Model file for the job. Use its own axes, mm. Face numbers are marked on the shaded views. A direction names the side the tool comes from. Coordinates: 2 decimals unless noted, no trailing zeros. Order: outer loops, then holes, each group sorted by start corner. A loop starts at its lowest first (then second) coordinate and runs counter-clockwise, first axis right, second up. Notation, with made-up numbers: (54, 62) -> (68, 62) arc R21 ccw to (68, 78) -> close; hole circle Ø8 at (42.5, -1.5). An arc over 180 degrees is marked (long way). Use CSV: the item, a comma, the result in double quotes. Start each with the question number.
(1) Cut at C-C on y = -13.5. Write the cut outline in (x, z) (3 decimals).
(2) Cut at B-B on x = 27.5. Write the cut outline in (y, z), plus the area to 3 significant figures.
(3) Pin check, flat tips, straight feed: pin 1 Ø1.5 at (x, y) = (16, -82) entering from +Z; pin 2 Ø0.7 at (x, y) = (14, -82) entering from -Z; pin 3 Ø9.5 at (x, y) = (21.5, -32) entering from -Z. Stop position of each tip, or through.
(4) Probe L1, parallel to Y at x = 30, z = 11; L2, parallel to Y at x = 16, z = 21.5 (3 decimals); L3, parallel to X at y = 15.5, z = 12. List the from-to ranges inside material, lowest first.
(5) Tool access for the marked faces 1, 2 and 3: list every direction of +Z, -Z, +X, -X, +Y, -Y with a clear straight run to the whole face (end or side of a thin tool).
(6) Pull direction X, two halves, no side cores. Call the marked faces 4, 5 and 6: pulls with the +X half, pulls with the -X half, needs draft (parallel to the pull), parting line crosses it, or undercut.
(7) Cut at A-A on z = 14. Write the cut outline in (x, y) (3 decimals), plus the area to 3 significant figures.
(8) Cut at D-D on z = 2.5. Write the cut outline in (x, y).
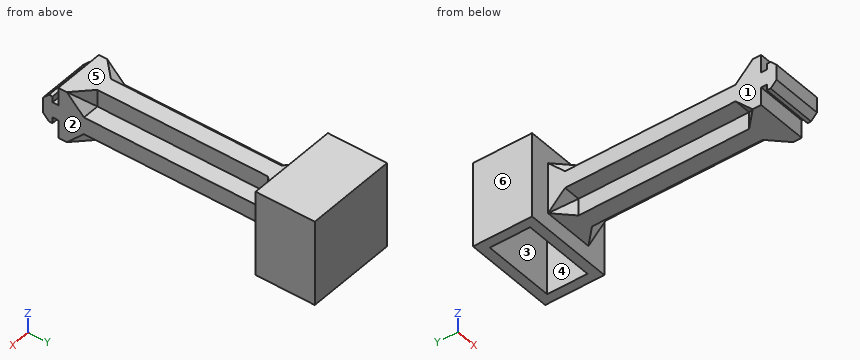
```python
from build123d import *

# Parameters (mm, degrees)
SKETCH1_W           = 34
SKETCH1_H           = 22
BOSS_EXTRUDE1_DEPTH = 31.75
SHELL1_T            = -3.5
BOSS_EXTRUDE2_DEPTH = 76.2
BOSS_EXTRUDE3_START = 26.525
BOSS_EXTRUDE3_DEPTH = 19.05
CHAMFER1_SIZE       = 6.35


with BuildPart() as part:
    # Sketch1 → Boss-Extrude1 (new body)
    with BuildSketch(Plane.XY):
        with Locations((17, 11)):
            Rectangle(SKETCH1_W, SKETCH1_H)
    extrude(amount=BOSS_EXTRUDE1_DEPTH)

    # Shell1
    shell1_openings = [part.faces().sort_by_distance(p)[0] for p in [
        (17, 11, 0),
    ]]
    offset(amount=SHELL1_T, openings=shell1_openings, kind=Kind.INTERSECTION)

    # Sketch2 → Boss-Extrude2 (add)
    with BuildSketch(Plane.XZ):
        Polygon((13.825, 25.189889706), (13.825, 18.839889706), (7.475, 18.839889706), (7.475, 12.489889706), (13.825, 12.489889706), (13.825, 6.139889706), (20.175, 6.139889706), (20.175, 12.489889706), (26.525, 12.489889706), (26.525, 18.839889706), (20.175, 18.839889706), (20.175, 25.189889706), align=None)
    extrude(amount=BOSS_EXTRUDE2_DEPTH)

    # Sketch3 → Boss-Extrude3 (add)
    with BuildSketch(Plane(origin=(0, 0, 0), x_dir=(0, 0, -1), z_dir=(1, 0, 0)).offset(BOSS_EXTRUDE3_START)):
        Polygon((-10.584889706, -81.534), (-10.584889706, -82.8675), (-12.807389706, -85.09), (-18.522389706, -85.09), (-20.744889706, -82.8675), (-20.744889706, -81.534), (-18.522389706, -81.534), (-18.522389706, -79.375), (-25.189889706, -79.375), (-25.189889706, -76.2), (-6.139889706, -76.2), (-6.139889706, -79.375), (-12.807389706, -79.375), (-12.807389706, -81.534), align=None)
    extrude(amount=-BOSS_EXTRUDE3_DEPTH)

    # Chamfer1
    # the kernel refuses this chamfer: 6.35 mm, written as the material it adds along each edge
    with BuildSketch(Plane(origin=(30.155186974, -76.2, 18.839889706), x_dir=(0, -0.027495876610585664, 0.9996219169112966), z_dir=(-1, 0, 0))) as chamfer1_piece_1_section:
        Polygon((CHAMFER1_SIZE * 0.999621916911, CHAMFER1_SIZE * 0.0274958766106), (-CHAMFER1_SIZE * 0.0274958766106, CHAMFER1_SIZE * 0.999621916911), (0, 0), align=None)
    chamfer1_piece_1 = extrude(amount=22.680186974, mode=Mode.PRIVATE)
    chamfer1_piece_1 = split(chamfer1_piece_1, bisect_by=Plane(origin=(26.525, -74.083333333, 20.956556373), z_dir=(-1, 0, 0)), keep=Keep.TOP, mode=Mode.PRIVATE)
    add(chamfer1_piece_1)
    with BuildSketch(Plane(origin=(13.825, -76.2, 25.189889706), x_dir=(-0.9996219169112966, -0.027495876610585654, 0), z_dir=(0, 0, -1))) as chamfer1_piece_2_section:
        Polygon((CHAMFER1_SIZE * 0.999621916911, CHAMFER1_SIZE * 0.0274958766106), (-CHAMFER1_SIZE * 0.0274958766106, CHAMFER1_SIZE * 0.999621916911), (0, 0), align=None)
    chamfer1_piece_2 = extrude(amount=22.680186974, mode=Mode.PRIVATE)
    chamfer1_piece_2 = split(chamfer1_piece_2, bisect_by=Plane(origin=(11.708333333, -74.083333333, 6.139889706), z_dir=(0, 0, 1)), keep=Keep.TOP, mode=Mode.PRIVATE)
    add(chamfer1_piece_2)
    with BuildSketch(Plane(origin=(26.525, -76.2, 18.839889706), x_dir=(0, -0.027495876610585654, 0.9996219169112968), z_dir=(-1, 0, 0))) as chamfer1_piece_3_section:
        Polygon((CHAMFER1_SIZE * 0.999621916911, CHAMFER1_SIZE * 0.0274958766106), (-CHAMFER1_SIZE * 0.0274958766106, CHAMFER1_SIZE * 0.999621916911), (0, 0), align=None)
    chamfer1_piece_3 = extrude(amount=22.680186974, mode=Mode.PRIVATE)
    chamfer1_piece_3 = split(chamfer1_piece_3, bisect_by=Plane(origin=(7.475, -74.083333333, 20.956556373), z_dir=(1, 0, 0)), keep=Keep.TOP, mode=Mode.PRIVATE)
    add(chamfer1_piece_3)
    with BuildSketch(Plane(origin=(20.175, -76.2, 2.509702732), x_dir=(0.9996219169112966, -0.02749587661058565, 0), z_dir=(0, 0, 1))) as chamfer1_piece_4_section:
        Polygon((CHAMFER1_SIZE * 0.999621916911, CHAMFER1_SIZE * 0.0274958766106), (-CHAMFER1_SIZE * 0.0274958766106, CHAMFER1_SIZE * 0.999621916911), (0, 0), align=None)
    chamfer1_piece_4 = extrude(amount=22.680186974, mode=Mode.PRIVATE)
    chamfer1_piece_4 = split(chamfer1_piece_4, bisect_by=Plane(origin=(22.291666667, -74.083333333, 6.139889706), z_dir=(0, 0, 1)), keep=Keep.TOP, mode=Mode.PRIVATE)
    add(chamfer1_piece_4)
    with BuildSketch(Plane(origin=(3.844813026, -76.2, 12.489889706), x_dir=(0, -0.027495876610585654, -0.9996219169112966), z_dir=(1, 0, 0))) as chamfer1_piece_5_section:
        Polygon((CHAMFER1_SIZE * 0.999621916911, CHAMFER1_SIZE * 0.0274958766106), (-CHAMFER1_SIZE * 0.0274958766106, CHAMFER1_SIZE * 0.999621916911), (0, 0), align=None)
    chamfer1_piece_5 = extrude(amount=22.680186974, mode=Mode.PRIVATE)
    chamfer1_piece_5 = split(chamfer1_piece_5, bisect_by=Plane(origin=(7.475, -74.083333333, 10.373223039), z_dir=(1, 0, 0)), keep=Keep.TOP, mode=Mode.PRIVATE)
    add(chamfer1_piece_5)
    with BuildSketch(Plane(origin=(20.175, -76.2, 6.139889706), x_dir=(0.9996219169112966, -0.02749587661058565, 0), z_dir=(0, 0, 1))) as chamfer1_piece_6_section:
        Polygon((CHAMFER1_SIZE * 0.999621916911, CHAMFER1_SIZE * 0.0274958766106), (-CHAMFER1_SIZE * 0.0274958766106, CHAMFER1_SIZE * 0.999621916911), (0, 0), align=None)
    chamfer1_piece_6 = extrude(amount=22.680186974, mode=Mode.PRIVATE)
    chamfer1_piece_6 = split(chamfer1_piece_6, bisect_by=Plane(origin=(22.291666667, -74.083333333, 25.189889706), z_dir=(0, 0, -1)), keep=Keep.TOP, mode=Mode.PRIVATE)
    add(chamfer1_piece_6)
    with BuildSketch(Plane(origin=(7.475, -76.2, 12.489889706), x_dir=(0, -0.027495876610585654, -0.9996219169112966), z_dir=(1, 0, 0))) as chamfer1_piece_7_section:
        Polygon((CHAMFER1_SIZE * 0.999621916911, CHAMFER1_SIZE * 0.0274958766106), (-CHAMFER1_SIZE * 0.0274958766106, CHAMFER1_SIZE * 0.999621916911), (0, 0), align=None)
    chamfer1_piece_7 = extrude(amount=22.680186974, mode=Mode.PRIVATE)
    chamfer1_piece_7 = split(chamfer1_piece_7, bisect_by=Plane(origin=(26.525, -74.083333333, 10.373223039), z_dir=(-1, 0, 0)), keep=Keep.TOP, mode=Mode.PRIVATE)
    add(chamfer1_piece_7)
    with BuildSketch(Plane(origin=(13.825, -76.2, 28.820076679), x_dir=(-0.9996219169112966, -0.02749587661058566, 0), z_dir=(0, 0, -1))) as chamfer1_piece_8_section:
        Polygon((CHAMFER1_SIZE * 0.999621916911, CHAMFER1_SIZE * 0.0274958766106), (-CHAMFER1_SIZE * 0.0274958766106, CHAMFER1_SIZE * 0.999621916911), (0, 0), align=None)
    chamfer1_piece_8 = extrude(amount=22.680186974, mode=Mode.PRIVATE)
    chamfer1_piece_8 = split(chamfer1_piece_8, bisect_by=Plane(origin=(11.708333333, -74.083333333, 25.189889706), z_dir=(0, 0, -1)), keep=Keep.TOP, mode=Mode.PRIVATE)
    add(chamfer1_piece_8)
    with BuildSketch(Plane(origin=(13.825, 0, 25.189889706), x_dir=(-0.9996219169112966, 0.02749587661058637, 0), z_dir=(0, 0, -1))) as chamfer1_piece_9_section:
        Polygon((CHAMFER1_SIZE * 0.999621916911, -CHAMFER1_SIZE * 0.0274958766106), (-CHAMFER1_SIZE * 0.0274958766106, -CHAMFER1_SIZE * 0.999621916911), (0, 0), align=None)
    chamfer1_piece_9 = extrude(amount=22.680186974, mode=Mode.PRIVATE)
    chamfer1_piece_9 = split(chamfer1_piece_9, bisect_by=Plane(origin=(11.708333333, -2.116666667, 6.139889706), z_dir=(0, 0, 1)), keep=Keep.TOP, mode=Mode.PRIVATE)
    add(chamfer1_piece_9)
    with BuildSketch(Plane(origin=(30.155186974, 0, 18.839889706), x_dir=(0, 0.027495876610586382, 0.9996219169112966), z_dir=(-1, 0, 0))) as chamfer1_piece_10_section:
        Polygon((CHAMFER1_SIZE * 0.999621916911, -CHAMFER1_SIZE * 0.0274958766106), (-CHAMFER1_SIZE * 0.0274958766106, -CHAMFER1_SIZE * 0.999621916911), (0, 0), align=None)
    chamfer1_piece_10 = extrude(amount=22.680186974, mode=Mode.PRIVATE)
    chamfer1_piece_10 = split(chamfer1_piece_10, bisect_by=Plane(origin=(26.525, -2.116666667, 20.956556373), z_dir=(-1, 0, 0)), keep=Keep.TOP, mode=Mode.PRIVATE)
    add(chamfer1_piece_10)
    with BuildSketch(Plane(origin=(26.525, 0, 18.839889706), x_dir=(0, -0.9996219169112966, -0.0274958766105862), z_dir=(-1, 0, 0))) as chamfer1_piece_11_section:
        Polygon((CHAMFER1_SIZE * 0.999621916911, CHAMFER1_SIZE * 0.0274958766106), (-CHAMFER1_SIZE * 0.0274958766106, CHAMFER1_SIZE * 0.999621916911), (0, 0), align=None)
    chamfer1_piece_11 = extrude(amount=22.680186974, mode=Mode.PRIVATE)
    chamfer1_piece_11 = split(chamfer1_piece_11, bisect_by=Plane(origin=(7.475, -2.116666667, 20.956556373), z_dir=(1, 0, 0)), keep=Keep.TOP, mode=Mode.PRIVATE)
    add(chamfer1_piece_11)
    with BuildSketch(Plane(origin=(20.175, 0, 2.509702732), x_dir=(-0.0274958766105862, -0.9996219169112966, 0), z_dir=(0, 0, 1))) as chamfer1_piece_12_section:
        Polygon((CHAMFER1_SIZE * 0.999621916911, CHAMFER1_SIZE * 0.0274958766106), (-CHAMFER1_SIZE * 0.0274958766106, CHAMFER1_SIZE * 0.999621916911), (0, 0), align=None)
    chamfer1_piece_12 = extrude(amount=22.680186974, mode=Mode.PRIVATE)
    chamfer1_piece_12 = split(chamfer1_piece_12, bisect_by=Plane(origin=(22.291666667, -2.116666667, 6.139889706), z_dir=(0, 0, 1)), keep=Keep.TOP, mode=Mode.PRIVATE)
    add(chamfer1_piece_12)
    with BuildSketch(Plane(origin=(20.175, 0, 6.139889706), x_dir=(0.9996219169112966, 0.027495876610586365, 0), z_dir=(0, 0, 1))) as chamfer1_piece_13_section:
        Polygon((CHAMFER1_SIZE * 0.999621916911, -CHAMFER1_SIZE * 0.0274958766106), (-CHAMFER1_SIZE * 0.0274958766106, -CHAMFER1_SIZE * 0.999621916911), (0, 0), align=None)
    chamfer1_piece_13 = extrude(amount=22.680186974, mode=Mode.PRIVATE)
    chamfer1_piece_13 = split(chamfer1_piece_13, bisect_by=Plane(origin=(22.291666667, -2.116666667, 25.189889706), z_dir=(0, 0, -1)), keep=Keep.TOP, mode=Mode.PRIVATE)
    add(chamfer1_piece_13)
    with BuildSketch(Plane(origin=(3.844813026, 0, 12.489889706), x_dir=(0, -0.9996219169112966, 0.02749587661058647), z_dir=(1, 0, 0))) as chamfer1_piece_14_section:
        Polygon((CHAMFER1_SIZE * 0.999621916911, CHAMFER1_SIZE * 0.0274958766106), (-CHAMFER1_SIZE * 0.0274958766106, CHAMFER1_SIZE * 0.999621916911), (0, 0), align=None)
    chamfer1_piece_14 = extrude(amount=22.680186974, mode=Mode.PRIVATE)
    chamfer1_piece_14 = split(chamfer1_piece_14, bisect_by=Plane(origin=(7.475, -2.116666667, 10.373223039), z_dir=(1, 0, 0)), keep=Keep.TOP, mode=Mode.PRIVATE)
    add(chamfer1_piece_14)
    with BuildSketch(Plane(origin=(13.825, 0, 28.820076679), x_dir=(-0.9996219169112966, 0.02749587661058637, 0), z_dir=(0, 0, -1))) as chamfer1_piece_15_section:
        Polygon((CHAMFER1_SIZE * 0.999621916911, -CHAMFER1_SIZE * 0.0274958766106), (-CHAMFER1_SIZE * 0.0274958766106, -CHAMFER1_SIZE * 0.999621916911), (0, 0), align=None)
    chamfer1_piece_15 = extrude(amount=22.680186974, mode=Mode.PRIVATE)
    chamfer1_piece_15 = split(chamfer1_piece_15, bisect_by=Plane(origin=(11.708333333, -2.116666667, 25.189889706), z_dir=(0, 0, -1)), keep=Keep.TOP, mode=Mode.PRIVATE)
    add(chamfer1_piece_15)
    with BuildSketch(Plane(origin=(7.475, 0, 12.489889706), x_dir=(0, 0.02749587661058637, -0.9996219169112966), z_dir=(1, 0, 0))) as chamfer1_piece_16_section:
        Polygon((CHAMFER1_SIZE * 0.999621916911, -CHAMFER1_SIZE * 0.0274958766106), (-CHAMFER1_SIZE * 0.0274958766106, -CHAMFER1_SIZE * 0.999621916911), (0, 0), align=None)
    chamfer1_piece_16 = extrude(amount=22.680186974, mode=Mode.PRIVATE)
    chamfer1_piece_16 = split(chamfer1_piece_16, bisect_by=Plane(origin=(26.525, -2.116666667, 10.373223039), z_dir=(-1, 0, 0)), keep=Keep.TOP, mode=Mode.PRIVATE)
    add(chamfer1_piece_16)


solid = part.part
```
Outcome:
1,outline,"(7.475, 12.49) -> (13.825, 12.49) -> (13.825, 6.14) -> (20.175, 6.14) -> (20.175, 12.49) -> (26.525, 12.49) -> (26.525, 18.84) -> (20.175, 18.84) -> (20.175, 25.19) -> (13.825, 25.19) -> (13.825, 18.84) -> (7.475, 18.84) -> close"
2,outline,"(0, 0) -> (3.5, 0) -> (3.5, 28.25) -> (18.5, 28.25) -> (18.5, 0) -> (22, 0) -> (22, 31.75) -> (0, 31.75) -> close"
2,area,"275 mm2"
3,pin 1,"z = 20.74"
3,pin 2,"z = 10.58"
3,pin 3,"z = 6.14"
4,L1,"0 to 3.5, 18.5 to 22"
4,L2,"-79.375 to 3.5, 18.5 to 22"
4,L3,"0 to 3.5, 30.5 to 34"
5,face 1,"+Z, -Z, -X, -Y"
5,face 2,"+Z, -Z, +X, -Y"
5,face 3,"-Z"
6,face 4,"undercut"
6,face 5,"needs draft"
6,face 6,"pulls with the -X half"
7,outline,"(0, 0) -> (7.475, 0) -> (7.475, -85.09) -> (26.525, -85.09) -> (26.525, 0) -> (34, 0) -> (34, 22) -> (0, 22) -> close; hole (3.5, 3.5) -> (30.5, 3.5) -> (30.5, 18.5) -> (3.5, 18.5) -> close"
7,area,"1,960 mm2"
8,outline,"(0, 0) -> (34, 0) -> (34, 22) -> (0, 22) -> close; hole (3.5, 3.5) -> (30.5, 3.5) -> (30.5, 18.5) -> (3.5, 18.5) -> close"
